Design review of the part built by this model. Coordinates are the model's own, in mm. Give positions to 0.01 mm unless a question says otherwise; leave off trailing zeros. Order: outer loops, then holes, each group sorted by start corner. A loop starts at its lowest first (then second) coordinate and runs counter-clockwise, first axis right, second up.
```python
from build123d import *

# Parameters (mm, degrees)
SKETCH1_R           = 2
SKETCH1_R_2         = 2.5
SKETCH1_R_3         = 5.5
SKETCH1_R_4         = 1.75
SKETCH1_R_5         = 8.75
SKETCH1_R_6         = 16
BOSS_EXTRUDE1_DEPTH = 3


with BuildPart() as part:
    # Sketch1 → Boss-Extrude1 (new body)
    with BuildSketch(Plane.XY):
        with BuildLine():
            ThreePointArc((-113.560266524, 49.479735972), (-130.694234864, 42.395842918), (-136.329525131, 24.732380193))
            ThreePointArc((-136.329525131, 24.732380193), (-137.686520221, 16.356467092), (-143.370984404, 10.056925608))
            ThreePointArc((-143.370984404, 10.056925608), (-155.166532009, -8.626129333), (-147.542861296, -29.364285714))
            ThreePointArc((-147.542861296, -29.364285714), (-143.475887893, -32.124161339), (-138.735140925, -33.421275181))
            ThreePointArc((-138.735140925, -33.421275181), (-127.733357788, -40.106373668), (-125.965715234, -52.858048609))
            ThreePointArc((-125.965715234, -52.858048609), (-121.095745986, -74.463536322), (-99.899442585, -80.88462828))
            Line((-99.899442585, -80.88462828), (87.590338172, -36.326384859))
            ThreePointArc((87.590338172, -36.326384859), (89.625170423, -35.311295666), (91, -33.5))
            ThreePointArc((91, -33.5), (97.213976906, 3.543991621), (84.648444567, 38.941424032))
            ThreePointArc((84.648444567, 38.941424032), (82.945648013, 40.504860181), (80.721588123, 41.135261877))
            Line((80.721588123, 41.135261877), (-113.560266524, 49.479735972))
        make_face()
        with Locations((-138.3, -22.75)):
            Circle(SKETCH1_R, mode=Mode.SUBTRACT)
        with Locations((-68.3, -21.5)):
            Circle(SKETCH1_R_2, mode=Mode.SUBTRACT)
        with Locations((-138.3, -5.25)):
            Circle(SKETCH1_R, mode=Mode.SUBTRACT)
        with Locations((-74.1, 1.7)):
            Circle(SKETCH1_R_2, mode=Mode.SUBTRACT)
        with Locations((18.7, -8.7)):
            Circle(SKETCH1_R_2, mode=Mode.SUBTRACT)
        with Locations((76.2, -22)):
            Circle(SKETCH1_R_2, mode=Mode.SUBTRACT)
        with Locations((8.2, 8.3)):
            Circle(SKETCH1_R_2, mode=Mode.SUBTRACT)
        with Locations((36.382449965, 0)):
            Circle(SKETCH1_R_3, mode=Mode.SUBTRACT)
        with Locations((78.2, -0.1)):
            Circle(SKETCH1_R_2, mode=Mode.SUBTRACT)
        with Locations((-112.981409671, 13.583075301)):
            Circle(SKETCH1_R_4, mode=Mode.SUBTRACT)
        with Locations((-128.421228626, 25.977105744)):
            Circle(SKETCH1_R_4, mode=Mode.SUBTRACT)
        with Locations((-65.3, 20)):
            Circle(SKETCH1_R_2, mode=Mode.SUBTRACT)
        with Locations((-114.504303927, 27.5)):
            Circle(SKETCH1_R_5, mode=Mode.SUBTRACT)
        with Locations((-100.587379227, 29.022894256)):
            Circle(SKETCH1_R_4, mode=Mode.SUBTRACT)
        with Locations((-116.027198182, 41.416924699)):
            Circle(SKETCH1_R_4, mode=Mode.SUBTRACT)
        with Locations((73.2, 22.3)):
            Circle(SKETCH1_R_2, mode=Mode.SUBTRACT)
        with Locations((-104.986214828, -59.480779371)):
            Circle(SKETCH1_R_6, mode=Mode.SUBTRACT)
    extrude(amount=BOSS_EXTRUDE1_DEPTH)


solid = part.part
```
1. Take a section at A-A (x = 8.2). State the section outline as (y, z) points, then the cut area to 3 significant figures.
Recorded:
outline: (-55.19, 0) - (5.8, 0) - (5.8, 3) - (-55.19, 3) - close; (10.8, 0) - (44.25, 0) - (44.25, 3) - (10.8, 3) - close
area: 283 mm2
2. Take a section at B-B (z = 1.4). State how many separate pieces and enclosed holes the cut face has, then the cut area to 3 significant figures.
Recorded:
separate pieces: 1
enclosed holes: 17
area: 23,300 mm2
3. For line 1 along X through (y, z) = (28, 2.8); line 2 along Y through (x, z) = (73.2, 1); line 3 along X through (y, z) = (-10.5, 1.8), list the stretches that pass through material, from the lowest coordinate up.
Recorded:
line 1: x = -136.5 to -123.24, -105.77 to -102.01, -99.17 to 90.78
line 2: y = -39.75 to 19.8, 24.8 to 41.46
line 3: x = -155.29 to 16.97, 20.43 to 97.12
4. Draft analysis for pull direction X (two halves, no side actions). For faces 1 (the face through (-116.78, -48.67, 1.48)), 2 (the face through (-67.8, 20.1, 1.5)), 3 (the face through (-155.13, -8.31, 1.48)), 4 (the face through (97.26, 3.01, 1.48)), state which applies: pulls with the +X half, pulls with the -X half, needs draft (parallel to the pull), parting line crosses it, or undercut.
Recorded:
face 1: undercut
face 2: undercut
face 3: pulls with the -X half
face 4: pulls with the +X half
5. For pin 1 (20 mm diameter, centred on x = -114.5, y = 27.5, fed in from -Z); pin 2 (1 mm diameter, centred on y = -53.5, z = 0.5, fed in from -X); pin 3 (2 mm diameter, centred on x = -128.42, y = 25.98, fed in from -Z); pin 4 (1.5 mm diameter, centred on y = -62, z = 2.5, fed in from -X), all flat-tipped, find the tip position at first contact; note any pin that passes through.
Recorded:
pin 1: stops at z = 0
pin 2: stops at x = -126.29
pin 3: passes through
pin 4: stops at x = -126.91
6. Take a section at C-C (x = 68). State the section outline as (y, z) points, then the cut area to 3 significant figures.
Recorded:
outline: (-40.98, 0) - (41.68, 0) - (41.68, 3) - (-40.98, 3) - close
area: 248 mm2
7. Take a section at D-D (x = -83). State the section outline as (y, z) points, then the cut area to 3 significant figures.
Recorded:
outline: (-76.87, 0) - (48.17, 0) - (48.17, 3) - (-76.87, 3) - close
area: 375 mm2
